```python
from build123d import *

# Parameters (mm, degrees)
BOSS_EXTRUDE1_DEPTH = 1210
SKETCH2_W           = 101.895059676
SKETCH2_H           = 138.127514373
CUT_EXTRUDE1_DEPTH  = 220


with BuildPart() as part:
    # Sketch1 → Boss-Extrude1 (new body)
    with BuildSketch(Plane(origin=(0, 0, 0), x_dir=(1, 0, 0), z_dir=(0, 1, 0))):
        with BuildLine():
            Line((-9, -10), (9, -10))
            ThreePointArc((9, -10), (9.707106781, -9.707106781), (10, -9))
            Line((10, -9), (10, 9))
            ThreePointArc((10, 9), (9.707106781, 9.707106781), (9, 10))
            Line((9, 10), (-9, 10))
            ThreePointArc((-9, 10), (-9.707106781, 9.707106781), (-10, 9))
            Line((-10, 9), (-10, -9))
            ThreePointArc((-10, -9), (-9.707106781, -9.707106781), (-9, -10))
        make_face()
        with BuildLine():
            Line((-7.5, -8.5), (7.5, -8.5))
            ThreePointArc((7.5, -8.5), (8.207106781, -8.207106781), (8.5, -7.5))
            Line((8.5, -7.5), (8.5, 7.5))
            ThreePointArc((8.5, 7.5), (8.207106781, 8.207106781), (7.5, 8.5))
            Line((7.5, 8.5), (-7.5, 8.5))
            ThreePointArc((-7.5, 8.5), (-8.207106781, 8.207106781), (-8.5, 7.5))
            Line((-8.5, 7.5), (-8.5, -7.5))
            ThreePointArc((-8.5, -7.5), (-8.207106781, -8.207106781), (-7.5, -8.5))
        make_face(mode=Mode.SUBTRACT)
    extrude(amount=BOSS_EXTRUDE1_DEPTH)

    # Sketch2 → Cut-Extrude1 (cut)
    with BuildSketch(Plane.XZ):
        with Locations((4.315799724, -16.6218454)):
            Rectangle(SKETCH2_W, SKETCH2_H)
    extrude(amount=-CUT_EXTRUDE1_DEPTH, mode=Mode.SUBTRACT)


solid = part.part
```
The model under review builds one solid part; all positions refer to its coordinate system, in mm. A direction names the side the tool comes from. Coordinates: 2 decimals unless noted, no trailing zeros. Write each loop counter-clockwise with the first axis right and the second up, starting at its lowest first coordinate (ties: lowest second). Pieces come first, ordered by that corner, then holes. Notation, with made-up numbers: (38, 38.5) - (77, 38.5) arc R19 cw to (77, 45.5) - close; hole circle Ø7 at (75.25, 22). An arc over 180 degrees is marked (long way). Answer in a Markdown table with one row per item. Add a question column.
Q1. Consider section C-C on x = -2. Give the boundary of the cut face in (y, z), then the cut area to 3 significant figures.
Q2. To check wall thickness, follow line 1 along X through (y, z) = (289, 2.75); line 2 along X through (y, z) = (931, -8). State the ranges of each line that lie inside material, in increasing order. Write a range as from..to.
Q3. Clearance check with a flat-ended pin moving along its axis: pin 1 (6 mm diameter, centred on x = 6.5, z = 7, fed in from -Y). State where the tip first meets the part, or that it passes through.
Q4. Consider section A-A on z = 2.5. Give the boundary of the cut face in (x, y), then the cut area to 3 significant figures.
Q5. Consider section B-B on y = 1026.5. Give the boundary of the cut face in (x, z), then the cut area to 3 significant figures.
Q6. For faces 1 (the face through (0, 708, -10)), 2 (the face through (8.5, 708, 0)), list the 3-axis set-ups (+Z, -Z, +X, -X, +Y, -Y) from which the entire face can be reached by the end or side of a thin tool; tool diameter is ignored.
Q7. Draft analysis for pull direction Z (two halves, no side actions). For faces 3 (the face through (0, 708, 10)), 4 (the face through (0, 708, -8.5)), 5 (the face through (-9, 1210, 0)), 6 (the face through (0, 708, 8.5)), state which applies: +Z half, -Z half, draft (parallel to the pull), parting line (faces both ways), or undercut.
Answers below:
| question | item | result |
|---|---|---|
| 1 | outline | (220, -10) - (1210, -10) - (1210, -8.5) - (220, -8.5) - close; (220, 8.5) - (1210, 8.5) - (1210, 10) - (220, 10) - close |
| 1 | area | 2,970 mm² |
| 2 | line 1 | -10..-8.5, 8.5..10 |
| 2 | line 2 | -10..-8.37, 8.37..10 |
| 3 | pin 1 | y = 220 |
| 4 | outline | (-10, 220) - (-8.5, 220) - (-8.5, 1210) - (-10, 1210) - close; (8.5, 220) - (10, 220) - (10, 1210) - (8.5, 1210) - close |
| 4 | area | 2,970 mm² |
| 5 | outline | (-10, -9) arc R1 ccw to (-9, -10) - (9, -10) arc R1 ccw to (10, -9) - (10, 9) arc R1 ccw to (9, 10) - (-9, 10) arc R1 ccw to (-10, 9) - close; hole (-8.5, -7.5) arc R1 ccw to (-7.5, -8.5) - (7.5, -8.5) arc R1 ccw to (8.5, -7.5) - (8.5, 7.5) arc R1 ccw to (7.5, 8.5) - (-7.5, 8.5) arc R1 ccw to (-8.5, 7.5) - close |
| 5 | area | 111 mm² |
| 6 | face 1 | -Z, +X, -X, +Y, -Y |
| 6 | face 2 | +Y, -Y |
| 7 | face 3 | +Z half |
| 7 | face 4 | undercut |
| 7 | face 5 | draft |
| 7 | face 6 | undercut |
